Source: CAD feature listing. Evaluate the final solid. Frame: model axes, mm. A direction names the side the tool comes from. Round coordinates to 2 decimals unless told otherwise and drop trailing zeros. Order: outer loops, then holes, each group sorted by start corner. A loop starts at its lowest first (then second) coordinate and runs counter-clockwise, first axis right, second up. Notation, with made-up numbers: (11.25, 17.25) - (57.25, 17.25) arc R27 ccw to (57.25, 52.25) - close; hole circle Ø7 at (-16.5, 86). An arc over 180 degrees is marked (long way). Use one line per item in the form item = value. Start each with the question number.
Q1. Cut plane D-D, the plane x = -5. Return the cut outline in (y, z).
Q2. Cut plane C-C, the plane y = 27. Return the cut outline in (x, z), and give its area (3 significant figures).
Q3. Cut plane B-B, the plane z = 2. Return the cut outline in (x, y), and give its area (3 significant figures).
Q4. Ray query, line 1 (Y direction, x = 0, z = 6.25); line 2 (Y direction, x = 3.5, z = 2.75); line 3 (X direction, y = 14, z = 3.75). Return the intervals inside material, ascending. Write a range as [from, to].
Q5. Cut plane A-A, the plane x = 0. Return the cut outline in (y, z).
Q6. Set-up query: faces 1 (the flat face through (0, 1, 10)), 2 (the flat face through (-2.8, -34.65, 1.48)), 3 (the flat face through (0, 30, 4)). Return all of +Z, -Z, +X, -X, +Y, -Y with unobstructed straight access to the full face (end or side cutting, diameter ignored); none if empty.
Q7. Pin query (flat end, axial travel): pin 1 Ø2.5 at (x, z) = (0, 1) entering from +Y; pin 2 Ø2 at (x, y) = (0, -48.5) entering from -Z. Return the tip coordinate at first contact, or that it passes through.
Q8. Draft query along Y for faces 4 (the flat face through (0, 5, 2)), 5 (the flat face through (-12.5, 30, 2)), 6 (the flat face through (0, -45.25, 1)). Return one class per face: released by +Y, released by -Y, zero draft, split by the parting line, or undercut.
from build123d import *

# Parameters (mm, degrees)
SKETCH1_W               = 29
SKETCH1_H               = 110
BOSS_EXTRUDE1_DEPTH     = 10
CUT_EXTRUDE1_DEPTH      = 112.401301608
CUT_EXTRUDE1_DEPTH_BACK = 50
SKETCH2_W               = 25
SKETCH2_H               = 4
SKETCH3_R               = 1.75
CUT_EXTRUDE2_DEPTH      = 58.751623354
CUT_EXTRUDE3_DEPTH      = 3


with BuildPart() as part:
    # Sketch1 → Boss-Extrude1 (new body)
    with BuildSketch(Plane.XY):
        Rectangle(SKETCH1_W, SKETCH1_H)
    extrude(amount=BOSS_EXTRUDE1_DEPTH)

    # Sketch2 → Cut-Extrude1 (cut, two sides: drawn at the far end of the back side and taken through both)
    with BuildSketch(Plane(origin=(0, 55, 0), x_dir=(1, 0, 0), z_dir=(0, 1, 0)).offset(-CUT_EXTRUDE1_DEPTH_BACK)):
        with Locations((0, -2)):
            Rectangle(SKETCH2_W, SKETCH2_H)
    extrude(amount=CUT_EXTRUDE1_DEPTH + CUT_EXTRUDE1_DEPTH_BACK, mode=Mode.SUBTRACT)

    # Sketch3 → Cut-Extrude2 (cut, through all)
    with BuildSketch(Plane(origin=(0, 0, 0), x_dir=(-1, 0, 0), z_dir=(0, 0, -1))):
        with Locations((0, -48.5)):
            Circle(SKETCH3_R)
        with Locations((0, -33)):
            Circle(SKETCH3_R)
    extrude(amount=-CUT_EXTRUDE2_DEPTH, mode=Mode.SUBTRACT)

    # Sketch5 → Cut-Extrude3 (cut)
    with BuildSketch(Plane(origin=(0, 0, 0), x_dir=(-1, 0, 0), z_dir=(0, 0, -1))):
        Polygon((1.876388375, -51.75), (3.75277675, -48.5), (1.876388375, -45.25), (-1.876388375, -45.25), (-3.75277675, -48.5), (-1.876388375, -51.75), align=None)
        Polygon((1.876388375, -36.25), (3.75277675, -33), (1.876388375, -29.75), (-1.876388375, -29.75), (-3.75277675, -33), (-1.876388375, -36.25), align=None)
    extrude(amount=-CUT_EXTRUDE3_DEPTH, mode=Mode.SUBTRACT)


solid = part.part
Completed:
q1.outline = (-55, 0) - (5, 0) - (5, 4) - (55, 4) - (55, 10) - (-55, 10) - close
q2.outline = (-14.5, 0) - (-12.5, 0) - (-12.5, 4) - (12.5, 4) - (12.5, 0) - (14.5, 0) - (14.5, 10) - (-14.5, 10) - close
q2.area = 190 mm2
q3.outline = (-14.5, -55) - (14.5, -55) - (14.5, 55) - (12.5, 55) - (12.5, 5) - (-12.5, 5) - (-12.5, 55) - (-14.5, 55) - close; hole (-3.75, -48.5) - (-1.88, -51.75) - (1.88, -51.75) - (3.75, -48.5) - (1.88, -45.25) - (-1.88, -45.25) - close; hole (-3.75, -33) - (-1.88, -36.25) - (1.88, -36.25) - (3.75, -33) - (1.88, -29.75) - (-1.88, -29.75) - close
q3.area = 1,870 mm2
q4.line_1 = [-55, -50.25], [-46.75, -34.75], [-31.25, 55]
q4.line_2 = [-55, -48.94], [-48.06, -33.44], [-32.56, 5]
q4.line_3 = [-14.5, -12.5], [12.5, 14.5]
q5.outline = (-55, 0) - (-51.75, 0) - (-51.75, 3) - (-50.25, 3) - (-50.25, 10) - (-55, 10) - close; (-46.75, 3) - (-45.25, 3) - (-45.25, 0) - (-36.25, 0) - (-36.25, 3) - (-34.75, 3) - (-34.75, 10) - (-46.75, 10) - close; (-31.25, 3) - (-29.75, 3) - (-29.75, 0) - (5, 0) - (5, 4) - (55, 4) - (55, 10) - (-31.25, 10) - close
q6.face_1 = +Z, +X, -X, +Y, -Y
q6.face_2 = -Z
q6.face_3 = -Z, +Y
q7.pin_1 = 5
q7.pin_2 = through
q8.face_4 = released by +Y
q8.face_5 = zero draft
q8.face_6 = undercut
